from build123d import *

# Parameters (mm, degrees)
SKETCH2_W           = 6.6
SKETCH2_H           = 2
BOSS_EXTRUDE1_DEPTH = 4
SKETCH3_W           = 5
SKETCH3_H           = 1.2
BOSS_EXTRUDE2_DEPTH = 4
SKETCH4_W           = 4
SKETCH4_H           = 1.2
BOSS_EXTRUDE3_DEPTH = 10
FILLET3_R           = 0.5


with BuildPart() as part:
    # Sketch2 → Boss-Extrude1 (new body)
    with BuildSketch(Plane(origin=(0, 0, 0), x_dir=(1, 0, 0), z_dir=(0, 1, 0))):
        Rectangle(SKETCH2_W, SKETCH2_H)
    extrude(amount=BOSS_EXTRUDE1_DEPTH)

    # Sketch3 → Boss-Extrude2 (add)
    with BuildSketch(Plane(origin=(0, 4, 0), x_dir=(1, 0, 0), z_dir=(0, 1, 0))):
        Rectangle(SKETCH3_W, SKETCH3_H)
    extrude(amount=BOSS_EXTRUDE2_DEPTH)

    # Sketch4 → Boss-Extrude3 (add)
    with BuildSketch(Plane(origin=(0, 8, 0), x_dir=(1, 0, 0), z_dir=(0, 1, 0))):
        Rectangle(SKETCH4_W, SKETCH4_H)
    extrude(amount=BOSS_EXTRUDE3_DEPTH)

    # Fillet3
    fillet3_edges = [part.edges().sort_by_distance(p)[0] for p in [
        (2.5, 8, 0),
        (-2.5, 8, 0),
        (2, 18, 0),
        (-2, 18, 0),
    ]]
    fillet(fillet3_edges, radius=FILLET3_R - 0.0001)  # a hair under: the kernel refuses the full size


solid = part.part
For this review, take the finished solid that the model builds, in its own axes (mm). A direction names the side the tool comes from. Give positions to 0.01 mm unless a question says otherwise; leave off trailing zeros. Loops run counter-clockwise (first coordinate to the right, second up) from the corner with the lowest first, then second, coordinate; pieces in that order, holes last.
Item 1: Take a section at C-C, the plane y = 6. State the section outline as (x, z) points, and give its area (3 significant figures).
Item 2: Take a section at D-D, the plane y = 15. State the section outline as (x, z) points.
Item 3: Tool access review of faces 1 (the flat face through (0, 11, -0.6)), 2 (the flat face through (2.5, 6, 0)), 3 (the flat face through (0, 11, 0.6)), 4 (the flat face through (-2, 13, 0)): name each direction out of +Z, -Z, +X, -X, +Y, -Y from which nothing blocks a thin tool from reaching the whole face with its end or side.
Item 4: Take a section at A-A, the plane x = -1.25. State the section outline as (y, z) points, and give its area (3 significant figures).
Item 5: Insertion check: pin 1 (3 mm diameter, centred on x = -1.5, y = 11.5, fed in from +Z); pin 2 (1.5 mm diameter, centred on x = 0.5, y = 14, fed in from -Z); pin 3 (0.6 mm diameter, centred on y = 5.5, z = 0, fed in from +X). Each pin has a flat end and moves straight along its axis. Give the tip position at first contact, or say it passes through.
Item 6: For line 1 along Y through (x, z) = (-1.75, 0.85); line 2 along X through (y, z) = (16.5, 0.4); line 3 along Z through (x, y) = (-1, 17), list the stretches that pass through material, from the lowest coordinate up.
Calculated:
1. outline: (-2.5, -0.6) - (2.5, -0.6) - (2.5, 0.6) - (-2.5, 0.6) - close
1. area: 6.00 mm2
2. outline: (-2, -0.6) - (2, -0.6) - (2, 0.6) - (-2, 0.6) - close
3. face 1: -Z, +X, -X, +Y
3. face 2: +Z, -Z, +X, +Y
3. face 3: +Z, +X, -X, +Y
3. face 4: +Z, -Z, -X, +Y
4. outline: (0, -1) - (4, -1) - (4, -0.6) - (18, -0.6) - (18, 0.6) - (4, 0.6) - (4, 1) - (0, 1) - close
4. area: 24.8 mm2
5. pin 1: stops at z = 0.6
5. pin 2: stops at z = -0.6
5. pin 3: stops at x = 2.5
6. line 1: y = 0 to 4
6. line 2: x = -2 to 2
6. line 3: z = -0.6 to 0.6
